Study the drawing (mm; zero at the part's minimum x, y, z) and answer. A direction names the side the tool comes from. Coordinates: 2 decimals unless noted, no trailing zeros. Order: outer loops, then holes, each group sorted by start corner. A loop starts at its lowest first (then second) coordinate and runs counter-clockwise, first axis right, second up. Notation, with made-up numbers: (13.5, -12.75) -> (46.5, -12.75) arc R19 ccw to (46.5, 18.25) -> close; hole circle Ø11 at (48, 65). An arc over 180 degrees is marked (long way). Answer as CSV lines item,"result". Start each with the question number.
Item 1: Section C-C (y = 39) is taken. Write down the section's boundary in (x, z).
Item 2: Each of these flat-tipped pins is pushed along its axis until it touches: pin 1 Ø2 at (y, z) = (59, 6.5) entering from +X; pin 2 Ø1 at (x, y) = (1.5, 61.5) entering from -Z; pin 3 Ø4 at (x, y) = (9.5, 66) entering from +Z; pin 4 Ø8 at (x, y) = (14, 58.5) entering from -Z. Where does it stop, or does it pass through?
Item 3: Section D-D (z = 15) is taken. Write down the section's boundary in (x, y), then the cut area to 3 significant figures.
Item 4: Section A-A (x = 8) is taken. Write down the section's boundary in (y, z).
Item 5: Section B-B (z = 8) is taken. Write down the section's boundary in (x, y).
Item 6: Straight lines are drawn through the part: L1, parallel to Y at x = 9.5, z = 14; L2, parallel to Z at x = 7.25, y = 43.5; L3, parallel to X at y = 41, z = 6.5. For each, find the intervals that lie inside material, in ascending order.
Item 7: Which of the six approach directions +Z, -Z, +X, -X, +Y, -Y give full straight-line access (tool end or side, diameter ignored) to the marked faces 1 and 2?
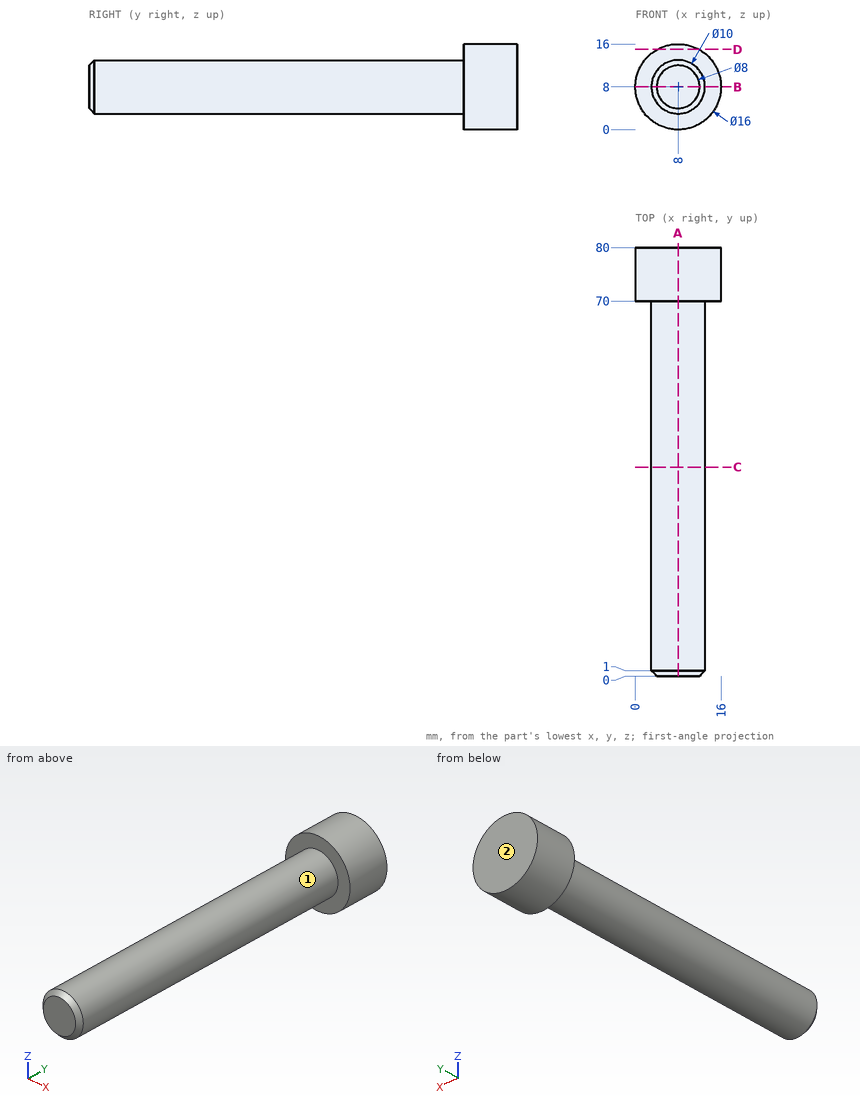
Checked values:
1,outline,"circle Ø10 at (8, 8)"
2,pin 1,"stops at x = 12.97"
2,pin 2,"passes through"
2,pin 3,"stops at z = 13"
2,pin 4,"stops at z = 3.42"
3,outline,"(4.13, 70) -> (11.87, 70) -> (11.87, 80) -> (4.13, 80) -> close"
3,area,"77.5 mm^2"
4,outline,"(0, 4) -> (1, 3) -> (70, 3) -> (70, 0) -> (80, 0) -> (80, 16) -> (70, 16) -> (70, 13) -> (1, 13) -> (0, 12) -> close"
5,outline,"(0, 70) -> (3, 70) -> (3, 1) -> (4, 0) -> (12, 0) -> (13, 1) -> (13, 70) -> (16, 70) -> (16, 80) -> (0, 80) -> close"
6,L1,"y = 70 to 80"
6,L2,"z = 3.06 to 12.94"
6,L3,"x = 3.23 to 12.77"
7,face 1,"-Y"
7,face 2,"+Z, -Z, +X, -X, +Y"
